```python
from build123d import *

# Parameters (mm, degrees)
CROQUIS1_R              = 3.175
SALIENTE_EXTRUIR1_DEPTH = 2.5


with BuildPart() as part:
    # Croquis1 → Saliente-Extruir1 (new, symmetric)
    with BuildSketch(Plane.XY):
        with BuildLine():
            Line((0, 0), (0, -50))
            ThreePointArc((0, -50), (5, -55), (10, -50))
            Line((10, -50), (10, 10))
            Line((10, 10), (-25, 10))
            ThreePointArc((-25, 10), (-30, 5), (-25, 0))
            Line((-25, 0), (0, 0))
        make_face()
        with Locations((5, -50)):
            Circle(CROQUIS1_R, mode=Mode.SUBTRACT)
        with Locations((5, 5)):
            Circle(CROQUIS1_R, mode=Mode.SUBTRACT)
        with Locations((-25, 5)):
            Circle(CROQUIS1_R, mode=Mode.SUBTRACT)
    extrude(amount=SALIENTE_EXTRUIR1_DEPTH, both=True)


solid = part.part
```
Geometry check sheet. Reference: the model listing, model coordinates, mm. A direction names the side the tool comes from. Coordinates: 2 decimals unless noted, no trailing zeros. Order: outer loops, then holes, each group sorted by start corner. A loop starts at its lowest first (then second) coordinate and runs counter-clockwise, first axis right, second up. Notation, with made-up numbers: (-32, 56.5) - (-26, 56.5) arc R16 cw to (-26, 64.5) - close; hole circle Ø8 at (87, 58). An arc over 180 degrees is marked (long way). Use one line per item in the form item = value.
1. Access from +Z, -Z, +X, -X, +Y, -Y to the whole of each face (thin tool, end or side, straight path). Record for faces 1 (the face through (-7, 10, 0)), 2 (the face through (-13, 0, 0)).
Here are the results:
face_1 = +Z, -Z, +X, -X, +Y
face_2 = +Z, -Z, -X, -Y
2. Section check A-A (x = 5). Record the boundary of the cut face in (y, z) (3 decimals).
Here are the results:
outline = (-55, -2.5) - (-53.175, -2.5) - (-53.175, 2.5) - (-55, 2.5) - close; (-46.825, -2.5) - (1.825, -2.5) - (1.825, 2.5) - (-46.825, 2.5) - close; (8.175, -2.5) - (10, -2.5) - (10, 2.5) - (8.175, 2.5) - close
3. Draft check along Y on faces 3 (the face through (5, -55, 0)), 4 (the face through (0, -25, 0)), 5 (the face through (4.31, -53.1, -0.04)). Enter one of: pulls with the +Y half, pulls with the -Y half, needs draft (parallel to the pull), parting line crosses it, or undercut.
Here are the results:
face_3 = pulls with the -Y half
face_4 = needs draft
face_5 = undercut
4. Scan lines: line 1 (Y direction, x = 5, z = -1.15) (3 decimals); line 2 (Y direction, x = -25, z = 0.9) (3 decimals); line 3 (Y direction, x = 6.5, z = 0.05). Record each from-to range of solid material in increasing order.
Here are the results:
line_1 = -55 to -53.175, -46.825 to 1.825, 8.175 to 10
line_2 = 0 to 1.825, 8.175 to 10
line_3 = -54.77 to -52.8, -47.2 to 2.2, 7.8 to 10
5. Section check D-D (y = -51). Record the boundary of the cut face in (x, z).
Here are the results:
outline = (0.1, -2.5) - (1.99, -2.5) - (1.99, 2.5) - (0.1, 2.5) - close; (8.01, -2.5) - (9.9, -2.5) - (9.9, 2.5) - (8.01, 2.5) - close
6. Section check B-B (z = 1.4). Record the boundary of the cut face in (x, y) (3 decimals).
Here are the results:
outline = (-25, 0) - (0, 0) - (0, -50) arc R5 ccw to (10, -50) - (10, 10) - (-25, 10) arc R5 ccw to start; hole circle Ø6.35 at (-25, 5); hole circle Ø6.35 at (5, -50); hole circle Ø6.35 at (5, 5)
7. Gauge pin test, flat ends, axial feed: pin 1 (5 mm diameter, centred on x = 5, y = -50, fed in from +Z); pin 2 (2.5 mm diameter, centred on y = -35.5, z = 0, fed in from -X); pin 3 (8.5 mm diameter, centred on x = -25, y = 5, fed in from -Z); pin 4 (2 mm diameter, centred on x = -20.5, z = -0.5, fed in from -Y). Record the tip position at first contact, or that the pin passes through.
Here are the results:
pin_1 = through
pin_2 = 0
pin_3 = -2.5
pin_4 = 0
8. Section check C-C (y = 5). Record the boundary of the cut face in (x, z) (3 decimals), then the cut area to 4 significant figures.
Here are the results:
outline = (-30, -2.5) - (-28.175, -2.5) - (-28.175, 2.5) - (-30, 2.5) - close; (-21.825, -2.5) - (1.825, -2.5) - (1.825, 2.5) - (-21.825, 2.5) - close; (8.175, -2.5) - (10, -2.5) - (10, 2.5) - (8.175, 2.5) - close
area = 136.5 mm²
